Check sheet for the drawn part. Datum: minimum x, y, z corner. Units: mm. A direction names the side the tool comes from. Coordinates: 2 decimals unless noted, no trailing zeros. Loops run counter-clockwise (first coordinate to the right, second up) from the corner with the lowest first, then second, coordinate; pieces in that order, holes last.
Q1. Go/stop test with flat-tipped pins: P1, Ø6.5, axis at y = 39.44, z = 10.61, coming from the +X side; P2, Ø8, axis at x = 5, z = 27, coming from the -Y side (1 decimal); P3, Ø3, axis at y = 20.5, z = 14.5, coming from the -X side. Record where each tip stops, or that it passes through.
Q2. Access from +Z, -Z, +X, -X, +Y, -Y to the whole of each face (thin tool, end or side, straight path). Record for the marked faces 4 and 5.
Q3. Sectioned sample at A-A (x = 10.75). Enter the section's corners in (y, z), then the cut area to 3 significant figures.
Q4. Sectioned sample at C-C (y = 22.5). Enter the section's corners in (x, z).
Q5. Sectioned sample at B-B (z = 25.5). Enter the section's corners in (x, y) (1 decimal).
Q6. Mould release check, pull along Y, two halves, no side actions. Record for the marked faces 1, 2 and 3: +Y half, -Y half, draft (parallel to the pull), parting line (faces both ways), or undercut.
Q7. Material ranges on probe 1 along Z at (x, y) = (13, 39.5); probe 2 along Y at (x, z) = (22.5, 30) (1 decimal); probe 3 along X at (y, z) = (31, 37), recorded low to high.
Q8. Sectioned sample at D-D (x = 22). Enter the section's corners in (y, z) (1 decimal), then the cut area to 3 significant figures.
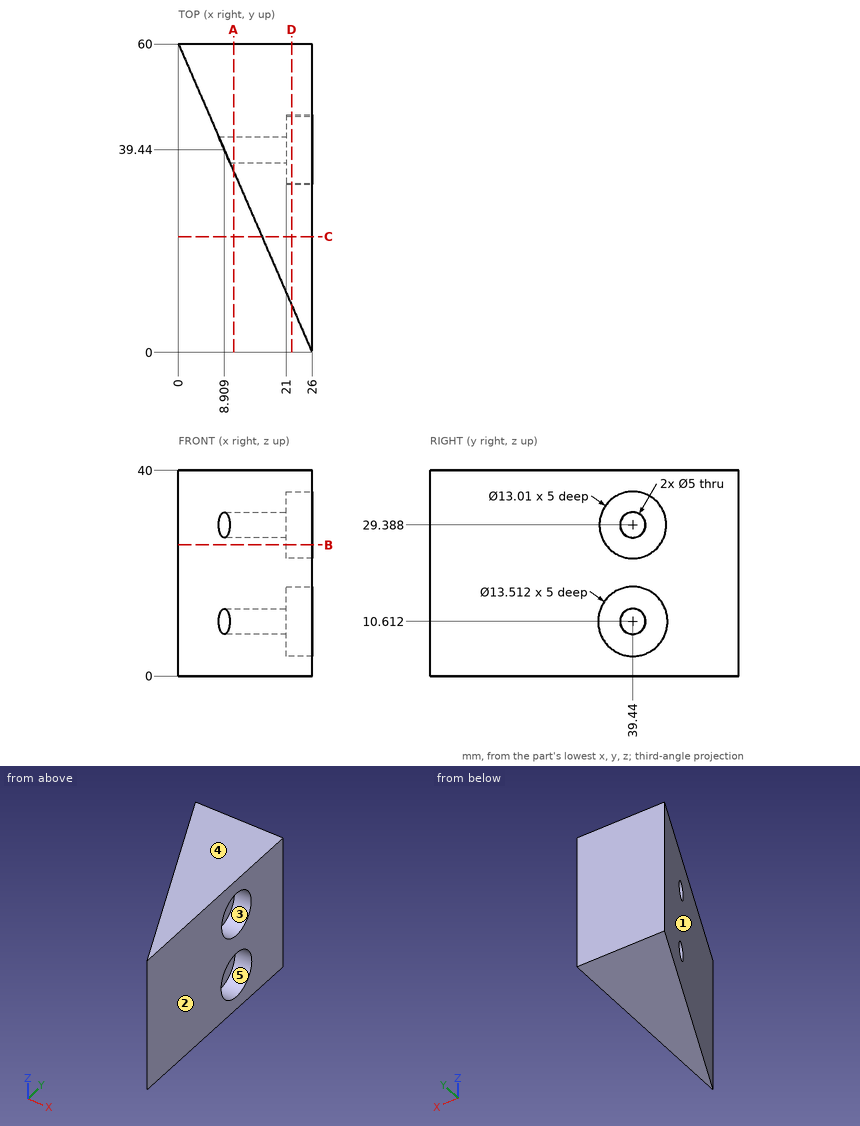
Geometry check:
1. P1: stops at x = 21
1. P2: stops at y = 39.2
1. P3: stops at x = 16.47
2. face 4: +Z, +X, -X, +Y, -Y
2. face 5: +X
3. outline: (35.19, 0) - (60, 0) - (60, 40) - (35.19, 40) - close; hole circle Ø5 at (39.44, 10.61); hole circle Ø5 at (39.44, 29.39)
3. area: 953 mm2
4. outline: (16.25, 0) - (26, 0) - (26, 40) - (16.25, 40) - close
5. outline: (0, 60) - (26, 0) - (26, 34.2) - (21, 34.2) - (21, 44.7) - (26, 44.7) - (26, 60) - close
6. face 1: -Y half
6. face 2: draft
6. face 3: undercut
7. probe 1: z = 0 to 8.11, 13.11 to 26.89, 31.89 to 40
7. probe 2: y = 8.1 to 33, 45.9 to 60
7. probe 3: x = 12.57 to 26
8. outline: (9.2, 0) - (60, 0) - (60, 40) - (9.2, 40) - close; hole circle Ø13.5 at (39.4, 10.6); hole circle Ø13 at (39.4, 29.4)
8. area: 1,750 mm2
